```python
from build123d import *

# Parameters (mm, degrees)
F0_W     = 101.6
F0_H     = 203.2
F1_DEPTH = 7.62
F3_DEPTH = 25.4
F4_W     = 12.7
F4_H     = 13.10565
F5_DEPTH = 101.6
F6_W     = 100
F6_H     = 50
F7_DEPTH = 12.954


with BuildPart() as f1:
    # F0 (on Top) → F1 (new body)
    with BuildSketch(Plane.XY):
        Rectangle(F0_W, F0_H)
    extrude(amount=F1_DEPTH)

    # F2 (on Top) → F3 (cut)
    with BuildSketch(Plane.XY):
        with BuildLine():
            Line((-15.035691, -77.822713), (-14.988321, -81.421245))
            ThreePointArc((-14.988321, -81.421245), (-13.081192, -83.592345), (-11.008666, -81.578528))
            Line((-11.008666, -81.578528), (-11.048887, -77.843856))
            ThreePointArc((-11.048887, -77.843856), (-13.031485, -75.796128), (-15.035691, -77.822713))
        make_face()
        with BuildLine():
            ThreePointArc((-15.035691, -95.377287), (-13.031485, -97.403872), (-11.048887, -95.356144))
            Line((-11.048887, -95.356144), (-11.008666, -91.621472))
            ThreePointArc((-11.008666, -91.621472), (-13.081192, -89.607655), (-14.988321, -91.778755))
            Line((-14.988321, -91.778755), (-15.035691, -95.377287))
        make_face()
        with BuildLine():
            ThreePointArc((15.035691, -77.822713), (13.031485, -75.796128), (11.048887, -77.843856))
            Line((11.048887, -77.843856), (11.008666, -81.578528))
            ThreePointArc((11.008666, -81.578528), (13.081192, -83.592345), (14.988321, -81.421245))
            Line((14.988321, -81.421245), (15.035691, -77.822713))
        make_face()
        with BuildLine():
            Line((11.008666, -91.621472), (11.048887, -95.356144))
            ThreePointArc((11.048887, -95.356144), (13.031485, -97.403872), (15.035691, -95.377287))
            Line((15.035691, -95.377287), (14.988321, -91.778755))
            ThreePointArc((14.988321, -91.778755), (13.081192, -89.607655), (11.008666, -91.621472))
        make_face()
        with BuildLine():
            ThreePointArc((15.035691, 95.377287), (13.031485, 97.403872), (11.048887, 95.356144))
            Line((11.048887, 95.356144), (11.008666, 91.621472))
            ThreePointArc((11.008666, 91.621472), (13.081192, 89.607655), (14.988321, 91.778755))
            Line((14.988321, 91.778755), (15.035691, 95.377287))
        make_face()
        with BuildLine():
            Line((-11.008666, 91.621472), (-11.048887, 95.356144))
            ThreePointArc((-11.048887, 95.356144), (-13.031485, 97.403872), (-15.035691, 95.377287))
            Line((-15.035691, 95.377287), (-14.988321, 91.778755))
            ThreePointArc((-14.988321, 91.778755), (-13.081192, 89.607655), (-11.008666, 91.621472))
        make_face()
        with BuildLine():
            ThreePointArc((-15.035691, 77.822713), (-13.031485, 75.796128), (-11.048887, 77.843856))
            Line((-11.048887, 77.843856), (-11.008666, 81.578528))
            ThreePointArc((-11.008666, 81.578528), (-13.081192, 83.592345), (-14.988321, 81.421245))
            Line((-14.988321, 81.421245), (-15.035691, 77.822713))
        make_face()
        with BuildLine():
            ThreePointArc((11.048887, 77.843856), (13.031485, 75.796128), (15.035691, 77.822713))
            Line((15.035691, 77.822713), (14.988321, 81.421245))
            ThreePointArc((14.988321, 81.421245), (13.081192, 83.592345), (11.008666, 81.578528))
            Line((11.008666, 81.578528), (11.048887, 77.843856))
        make_face()
    extrude(amount=F3_DEPTH, mode=Mode.SUBTRACT)

    # F4 (on face) → F5 (join)
    with BuildSketch(Plane.XY.offset(7.62)):
        with Locations((38.1, 88.9)):
            Rectangle(F4_W, F4_H)
        with Locations((-38.1, 88.9)):
            Rectangle(F4_W, F4_H)
        with Locations((38.1, -88.9)):
            Rectangle(F4_W, F4_H)
        with Locations((-38.1, -88.9)):
            Rectangle(F4_W, F4_H)
    extrude(amount=F5_DEPTH)

    # F6 (on face) → F7 (join)
    with BuildSketch(Plane.XY.offset(7.62)):
        Polygon((50, 25.5842), (-50, 25.5842), (-50.777242, 25), (-50.777242, -25), (-50, -25.5842), (50, -25.5842), (50.762001, -25), (50.762001, 25), align=None)
        Rectangle(F6_W, F6_H, mode=Mode.SUBTRACT)
    extrude(amount=F7_DEPTH)


solid = f1.part
```
CAD build for the part. Positions are in the model's coordinates, mm. A direction names the side the tool comes from. Give positions to 0.01 mm unless a question says otherwise; leave off trailing zeros. Order: outer loops, then holes, each group sorted by start corner. A loop starts at its lowest first (then second) coordinate and runs counter-clockwise, first axis right, second up.
(1) Tool access for faces 1 (the flat face through (-1, 1, 0)), 2 (the flat face through (-1, -25.584, 14)), 3 (the cylindrical face through (13.036, 89.606, 3.757)): list every direction of +Z, -Z, +X, -X, +Y, -Y with a clear straight run to the whole face (end or side of a thin tool).
(2) Flat gauge pins, fed straight in: pin 1 (10.5 mm diameter, centred on y = 91, z = 44, fed in from -X); pin 2 (6 mm diameter, centred on x = -26.5, y = 0, fed in from +Z); pin 3 (4 mm diameter, centred on x = 13.5, z = 14, fed in from +Y); pin 4 (12 mm diameter, centred on y = -74.5, z = 63, fed in from -X). Where does each tip first touch, or does it go through?
(3) Saw through at B-B, the plane z = 91.5. Give the cut face in (x, y).
(4) Mould opens along Y. For faces 4 (the flat face through (50, 0, 14)), 5 (the flat face through (-1, 101.6, 4)), 6 (the cylindrical face through (-13.076, 75.796, 3.757)), 7 (the flat face through (-50.8, -1, 4)) say: released by +Y, released by -Y, zero draft, split by the parting line, or undercut.
(5) Drill centre lines: L1, parallel to Y at x = -36.5, z = 8.5; L2, parallel to Y at x = -42, z = 92.5; L3, parallel to X at y = 24, z = 10.5. Where is each one in solid material? Low to high.
(6) Saw through at D-D, the plane x = -19.5. Give the cut face in (y, z).
(7) Saw through at A-A, the plane z = 12. Give the cut face in (x, y), then the cut area to 3 significant figures.
Results found:
1. face 1: -Z, +X, -X, +Y, -Y
1. face 2: +Z, +X, -X
1. face 3: +Z, -Z
2. pin 1: stops at x = -44.45
2. pin 2: stops at z = 7.62
2. pin 3: stops at y = 25.58
2. pin 4: passes through
3. outline: (-44.45, -95.45) - (-31.75, -95.45) - (-31.75, -82.35) - (-44.45, -82.35) - close; (-44.45, 82.35) - (-31.75, 82.35) - (-31.75, 95.45) - (-44.45, 95.45) - close; (31.75, -95.45) - (44.45, -95.45) - (44.45, -82.35) - (31.75, -82.35) - close; (31.75, 82.35) - (44.45, 82.35) - (44.45, 95.45) - (31.75, 95.45) - close
4. face 4: undercut
4. face 5: released by +Y
4. face 6: undercut
4. face 7: zero draft
5. L1: y = -95.45 to -82.35, -25.58 to -25, 25 to 25.58, 82.35 to 95.45
5. L2: y = -95.45 to -82.35, 82.35 to 95.45
5. L3: x = -50.78 to -50, 50 to 50.76
6. outline: (-101.6, 0) - (101.6, 0) - (101.6, 7.62) - (25.58, 7.62) - (25.58, 20.57) - (25, 20.57) - (25, 7.62) - (-25, 7.62) - (-25, 20.57) - (-25.58, 20.57) - (-25.58, 7.62) - (-101.6, 7.62) - close
7. outline: (-50.78, -25) - (-50, -25.58) - (50, -25.58) - (50.76, -25) - (50.76, 25) - (50, 25.58) - (-50, 25.58) - (-50.78, 25) - close; (-44.45, -95.45) - (-31.75, -95.45) - (-31.75, -82.35) - (-44.45, -82.35) - close; (-44.45, 82.35) - (-31.75, 82.35) - (-31.75, 95.45) - (-44.45, 95.45) - close; (31.75, -95.45) - (44.45, -95.45) - (44.45, -82.35) - (31.75, -82.35) - close; (31.75, 82.35) - (44.45, 82.35) - (44.45, 95.45) - (31.75, 95.45) - close; hole (-50, -25) - (50, -25) - (50, 25) - (-50, 25) - close
7. area: 860 mm2
